Verification items for the finished model (mm, model axes). A direction names the side the tool comes from. Coordinates: 2 decimals unless noted, no trailing zeros. Write each loop counter-clockwise with the first axis right and the second up, starting at its lowest first coordinate (ties: lowest second). Pieces come first, ordered by that corner, then holes.
```python
from build123d import *

# Parameters (mm, degrees)
F0_R          = 29
F1_DEPTH      = 10
F2_R          = 29
F2_R_2        = 16
F3_DEPTH      = 5
F4_SIZE       = 4
F5_T          = -1
F6_R          = 1.5
F7_DEPTH      = 1.5
F8_W          = 5
F8_H          = 1
F9_DEPTH      = 29.001
F9_DEPTH_BACK = 29.001


with BuildPart() as f1:
    # F0 (on Top) → F1 (new body)
    with BuildSketch(Plane.XY):
        Circle(F0_R)
    extrude(amount=F1_DEPTH)

    # F2 (on face) → F3 (cut)
    with BuildSketch(Plane(origin=(0, 0, 0), x_dir=(1, 0, 0), z_dir=(0, 0, -1))):
        Circle(F2_R)
        Circle(F2_R_2, mode=Mode.SUBTRACT)
    extrude(amount=-F3_DEPTH, mode=Mode.SUBTRACT)

    # F4
    f4_edges = [f1.edges().sort_by_distance(p)[0] for p in [
        (-16, 0, 5),
    ]]
    chamfer(f4_edges, length=F4_SIZE)

    # F5
    f5_openings = [f1.faces().sort_by_distance(p)[0] for p in [
        (0, 0, 10),
        (0, 0, 0),
    ]]
    offset(amount=F5_T, openings=f5_openings, kind=Kind.INTERSECTION)

    # F6 (on face) → F7 (join)
    with BuildSketch(Plane.XY.offset(6)):
        with Locations((-24, 0)):
            Circle(F6_R)
        with Locations((24, 0)):
            Circle(F6_R)
    extrude(amount=F7_DEPTH)

    # F8 (on Front) → F9 (cut, two sides)
    with BuildSketch(Plane.XZ) as f9_sk:
        with Locations((0, 0.5)):
            Rectangle(F8_W, F8_H)
    extrude(amount=-F9_DEPTH, mode=Mode.SUBTRACT)
    extrude(f9_sk.sketch, amount=F9_DEPTH_BACK, mode=Mode.SUBTRACT)


solid = f1.part
```
1. Sectioned sample at D-D, the plane y = 25. Record the boundary of the cut face in (x, z).
2. Material ranges on L1, parallel to X at y = 0, z = 0.4; L2, parallel to Y at x = 0, z = 7.35; L3, parallel to Z at x = 15.5, y = -15.5, recorded low to high.
3. Tool access check on faces 1 (the cylindrical face through (15.997, 0.317, 0.493)), 2 (the flat face through (24, 0, 7.5)), 3 (the cylindrical face through (-15.997, -0.317, 0.493)), 4 (the flat face through (-7, 19, 5)). Record the directions out of +Z, -Z, +X, -X, +Y, -Y that give a thin tool (end or side, any length) a straight path to the whole face; none if there is none.
4. Sectioned sample at B-B, the plane x = 0. Record the boundary of the cut face in (y, z), and give its area (3 significant figures).
5. Draft check along Y on faces 5 (the flat face through (-15, 24, 10)), 6 (the cylindrical face through (-3.252, 14.643, 0.697)), 7 (the cylindrical face through (13.38, -25.73, 7.46)). Enter one of: pulls with the +Y half, pulls with the -Y half, needs draft (parallel to the pull), parting line crosses it, or undercut.
6. Sectioned sample at A-A, the plane y = 0. Record the boundary of the cut face in (x, z).
7. Gauge pin test, flat ends, axial feed: P1, Ø1.1, axis at y = 15, z = 0.5, coming from the -X side; P2, Ø0.6, axis at x = 1, y = 15, coming from the -Z side; P3, Ø4, axis at x = 8.5, z = 7.5, coming from the +Y side. Record the tip position at first contact, or that the pin passes through.
8. Sectioned sample at C-C, the plane z = 8.5. Record the boundary of the cut face in (x, y), and give its area (3 significant figures).
Outcome:
1. outline: (-14.7, 5) - (14.7, 5) - (14.7, 10) - (12.61, 10) - (12.61, 6) - (-12.61, 6) - (-12.61, 10) - (-14.7, 10) - close
2. L1: x = -16 to -15, 15 to 16
2. L2: y = -29 to -28, 28 to 29
2. L3: z = 5 to 6
3. face 1: -Z, +X
3. face 2: +Z
3. face 3: -Z, -X
3. face 4: -Z
4. outline: (-29, 5) - (-20, 5) - (-16, 1) - (-15, 1) - (-15, 1.41) - (-19.59, 6) - (-28, 6) - (-28, 10) - (-29, 10) - close; (15, 1) - (16, 1) - (20, 5) - (29, 5) - (29, 10) - (28, 10) - (28, 6) - (19.59, 6) - (15, 1.41) - close
4. area: 39.0 mm2
5. face 5: needs draft
5. face 6: undercut
5. face 7: parting line crosses it
6. outline: (-29, 5) - (-20, 5) - (-16, 1) - (-16, 0) - (-15, 0) - (-15, 1.41) - (-19.59, 6) - (-22.5, 6) - (-22.5, 7.5) - (-25.5, 7.5) - (-25.5, 6) - (-28, 6) - (-28, 10) - (-29, 10) - close; (15, 0) - (16, 0) - (16, 1) - (20, 5) - (29, 5) - (29, 10) - (28, 10) - (28, 6) - (25.5, 6) - (25.5, 7.5) - (22.5, 7.5) - (22.5, 6) - (19.59, 6) - (15, 1.41) - close
7. P1: stops at x = -6.87
7. P2: stops at z = 1
7. P3: stops at y = 28.26
8. outline: circle Ø58 at (0, 0); hole circle Ø56 at (0, 0)
8. area: 179 mm2
